Autodesk Inventor part; units mm, degrees
ref_plane "YZ Plane" through (0, 0, 0) normal (1, 0, 0) x (0, 1, 0)
ref_plane "XZ Plane" through (0, 0, 0) normal (0, 1, 0) x (-1, 0, 0)
ref_plane "XY Plane" through (0, 0, 0) normal (0, 0, 1) x (1, 0, 0)
sketch "Esboço2" plane through (0, 0, 0) normal (0, 1, 0) x (-1, 0, 0)
  circle A0 centre (3.8014, 2.7994) radius 1.25
  circle A1 centre (-3.8014, -2.7994) radius 1.25
  arc A2 (-5, 5) -> (-6, 4) centre (-5, 4) ccw
  line L0 (-6, 4) -> (-6, -4)
  arc A3 (-6, -4) -> (-5, -5) centre (-5, -4) ccw
  line L1 (-5, -5) -> (5, -5)
  arc A4 (5, -5) -> (6, -4) centre (5, -4) ccw
  line L2 (6, -4) -> (6, 4)
  arc A5 (6, 4) -> (5, 5) centre (5, 4) ccw
  line L3 (5, 5) -> (-5, 5)
  circle A6 centre (0, 0) radius 2
  arc A7 (0.45, -5) -> (-0.45, -5) centre (0, -5) ccw
  circle A8 centre (3.8014, 2.7994) radius 0.75
  circle A9 centre (-3.8014, -2.7994) radius 0.75
  circle A10 centre (-3.0146, 1.9633) radius 0.45
  circle A11 centre (0, 3) radius 0.45
  line L4 (0, 0) -> (0, 5)
  dimension "d16" = 0.9
  dimension "d17" = 1.5
  dimension "d18" = 1.5
  dimension "d23" = 4
  dimension "d26" = 2
  dimension "d27" = 0
extrude "Extrusão3" add sketch "Esboço2" along normal blind 0.8 contours A11 L4 | L4 A11 | L3 A5 L2 A4 L1 A7 A3 L0 A2 | A10
extrude "Extrusão4" add sketch "Esboço2" along normal blind 0.4 contours A0 | A1
extrude "Extrusão5" cut sketch "Esboço2" along normal blind 10 contours A10
extrude "Extrusão6" cut sketch "Esboço2" along normal blind 10 contours A11 L4 | L4 A11
sketch "Esboço4" plane through (0, 0.8, 0) normal (0, 1, 0) x (1, 0, 0)
  point P0 (0, 0)
properties part number "Chapa Inferior"
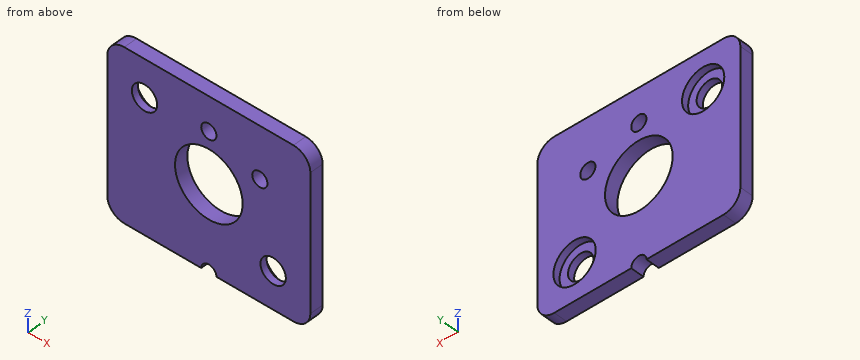
Geometry: final body of the model. Coordinates: model frame, mm. Round coordinates to 2 decimals unless told otherwise and drop trailing zeros. Order: outer loops, then holes, each group sorted by start corner. A loop starts at its lowest first (then second) coordinate and runs counter-clockwise, first axis right, second up. Notation, with made-up numbers: (10, 44.5) - (68, 44.5) arc R22 cw to (68, 53.5) - close; hole circle Ø1 at (-6.5, 40.5). An arc over 180 degrees is marked (long way). Use CSV: the item, a comma, the result in double quotes. Start each with the question number.
Q1. Section query B-B (x = 0). Return loops of the section in (y, z).
Q2. Section query D-D (y = 0.55). Return loops of the section in (x, z), and give its area (3 significant figures).
Q3. First-contact query: pin 1 (1.2 mm diameter, centred on x = -4, z = 3, fed in from +Y). Flat tip, straight axial feed; report the tip coordinate or a pass-through.
Q4. Material intervals for line 1 along Z through (x, y) = (0, 0.6); line 2 along Z through (x, y) = (2.75, 0.5); line 3 along Y through (x, z) = (4.5, -2), sorted ascending. Write a range as from..to.
Q5. Section query A-A (z = 0). Return loops of the section in (x, y).
Q6. Section query C-C (x = 4). Return loops of the section in (y, z), and give its area (3 significant figures).
Result set:
1,outline,"(0, -4.55) - (0.8, -4.55) - (0.8, -2) - (0, -2) - close; (0, 2) - (0.8, 2) - (0.8, 2.55) - (0, 2.55) - close; (0, 3.45) - (0.8, 3.45) - (0.8, 5) - (0, 5) - close"
2,outline,"(-6, -4) arc R1 ccw to (-5, -5) - (-0.45, -5) arc R0.45 cw to (0.45, -5) - (5, -5) arc R1 ccw to (6, -4) - (6, 4) arc R1 ccw to (5, 5) - (-5, 5) arc R1 ccw to (-6, 4) - close; hole circle Ø2.5 at (-3.8, 2.8); hole circle Ø4 at (0, 0); hole circle Ø0.9 at (0, 3); hole circle Ø2.5 at (3.8, -2.8); hole circle Ø0.9 at (3.01, 1.96)"
2,area,"95.2 mm2"
3,pin 1,"stops at y = 0.4"
4,line 1,"z = -4.55..-2, 2..2.55, 3.45..5"
4,line 2,"z = -5..-3.48, -2.12..1.6, 2.33..5"
4,line 3,"y = 0..0.4"
5,outline,"(-6, 0) - (-2, 0) - (-2, 0.8) - (-6, 0.8) - close; (2, 0) - (6, 0) - (6, 0.8) - (2, 0.8) - close"
6,outline,"(0, -5) - (0.8, -5) - (0.8, -4.03) - (0.4, -4.03) - (0.4, -3.52) - (0, -3.52) - close; (0, -2.08) - (0.4, -2.08) - (0.4, -1.57) - (0.8, -1.57) - (0.8, 5) - (0, 5) - close"
6,area,"6.43 mm2"
